Can you work these out from the model? Positions are in its coordinate system, mm. Face numbers are marked on the shaded views. A direction names the side the tool comes from. Round coordinates to 2 decimals unless told otherwise and drop trailing zeros. Loops run counter-clockwise (first coordinate to the right, second up) from the corner with the lowest first, then second, coordinate; pieces in that order, holes last. Notation, with made-up numbers: M -12,65.5 L 4,65.5 A33 ccw 4,93.5 Z; hole C 53.25,28 d7. An arc over 180 degrees is marked long. Answer as CSV lines item,"result".
from build123d import *

# Parameters (mm, degrees)
MAINBASESKETCH_W              = 47.8
MAINBASESKETCH_H              = 3.2
MAINBASEEXTRUDE_DEPTH         = 7.9
MAINBASESHELL_T               = -1.2
UNDERSIDECIRCLEEXT_START      = -0.2
UNDERSIDECIRCLESKETCH_R       = 3.25
UNDERSIDECIRCLESKETCH_R_2     = 2.4
UNDERSIDECIRCLEEXT_DEPTH      = 2.4
UNDERSIDECIRCLEPATTERN_COUNT  = 2
UNDERSIDECIRCLEPATTERN_PITCH  = 8
EXTENDEDBASEEDGECUT_DEPTH     = 0.2
EXTENDEDBASEEDGECUT2_DEPTH    = 0.2
EXTENDEDBASEEDGECUT3_DEPTH    = 0.2
EXTENDEDBASEEDGESKETCH4_W     = 47.4
EXTENDEDBASEEDGESKETCH4_H     = 0.199766916
EXTENDEDBASEEDGECUT4_DEPTH    = 0.2
EXTENDEDNBASEUNDERNOTCH_DEPTH = 0.4
EXTENDEBASENOTCHFILLET_R      = 0.2
CUT_EXTRUDE61_DEPTH           = 50.22551315
CUT_EXTRUDE61_DEPTH_BACK      = 50.22551315


with BuildPart() as part:
    # MainBaseSketch → MainBaseExtrude (new, symmetric)
    with BuildSketch(Plane.XY):
        with Locations((24.581967213, 1.6)):
            Rectangle(MAINBASESKETCH_W, MAINBASESKETCH_H)
    extrude(amount=MAINBASEEXTRUDE_DEPTH, both=True)

    # MainBaseShell
    mainbaseshell_openings = [part.faces().sort_by_distance(p)[0] for p in [
        (24.581967213, 0, 0),
    ]]
    offset(amount=MAINBASESHELL_T, openings=mainbaseshell_openings, kind=Kind.INTERSECTION)

    # UnderSideCircleSketch → UnderSideCircleExt (add)
    with BuildSketch(Plane.XZ.offset(-2).offset(UNDERSIDECIRCLEEXT_START)):
        with Locations((8.581967213, 0)):
            Circle(UNDERSIDECIRCLESKETCH_R)
        with Locations((8.581967213, 0)):
            Circle(UNDERSIDECIRCLESKETCH_R_2, mode=Mode.SUBTRACT)
    undersidecircleext = extrude(amount=UNDERSIDECIRCLEEXT_DEPTH)

    # UnderSideCirclePattern: UnderSideCircleExt ×2
    with Locations(*[(i * UNDERSIDECIRCLEPATTERN_PITCH, 0, 0) for i in range(1, UNDERSIDECIRCLEPATTERN_COUNT)]):
        add(undersidecircleext)

    # ExtendedBaseEdgeSketch → ExtendedBaseEdgeCut (cut)
    with BuildSketch(Plane.ZY.offset(-0.681967213)):
        Polygon((-7.9, 0), (-7.9, 0.199766916), (-7.702184024, 0.199766916), (7.702184024, 0.199766916), (7.9, 0.199766916), (7.9, 0), (7.702184024, 0), (-7.702184024, 0), align=None)
    extrude(amount=-EXTENDEDBASEEDGECUT_DEPTH, mode=Mode.SUBTRACT)

    # ExtendedBaseEdgeSketch2 → ExtendedBaseEdgeCut2 (cut)
    with BuildSketch(Plane(origin=(0, 0, -7.9), x_dir=(-1, 0, 0), z_dir=(0, 0, -1))):
        Polygon((-48.481967213, 0), (-48.481967213, 0.203418418), (-0.881967213, 0.199766916), (-0.881967213, 0), align=None)
    extrude(amount=-EXTENDEDBASEEDGECUT2_DEPTH, mode=Mode.SUBTRACT)

    # ExtendedBaseEdgeSketch3 → ExtendedBaseEdgeCut3 (cut)
    with BuildSketch(Plane(origin=(48.481967213, 0, 0), x_dir=(0, 0, -1), z_dir=(1, 0, 0))):
        Polygon((-7.9, 0), (-7.9, 0.199766916), (7.7, 0.203418418), (7.7, 0), align=None)
    extrude(amount=-EXTENDEDBASEEDGECUT3_DEPTH, mode=Mode.SUBTRACT)

    # ExtendedBaseEdgeSketch4 → ExtendedBaseEdgeCut4 (cut)
    with BuildSketch(Plane.XY.offset(7.9)):
        with Locations((24.581967213, 0.099883458)):
            Rectangle(EXTENDEDBASEEDGESKETCH4_W, EXTENDEDBASEEDGESKETCH4_H)
    extrude(amount=-EXTENDEDBASEEDGECUT4_DEPTH, mode=Mode.SUBTRACT)

    # ExtendedbaseUnderNotchSketch → ExtendednbaseUnderNotch (cut)
    with BuildSketch(Plane.XZ.offset(-2)):
        Polygon((1.881967213, 0), (1.881967213, 2.502100162), (2.381942481, 2.502100162), (2.381942481, -2.499482153), (1.881967213, -2.499482153), align=None)
    extrude(amount=-EXTENDEDNBASEUNDERNOTCH_DEPTH, mode=Mode.SUBTRACT)

    # ExtendebaseNotchFillet
    extendebasenotchfillet_edges = [part.edges().sort_by_distance(p)[0] for p in [
        (1.881967213, 2.4, 0.001309004),
        (2.131954847, 2.4, 2.502100162),
        (2.381942481, 2.4, 0.001309004),
        (2.131954847, 2.4, -2.499482153),
    ]]
    fillet(extendebasenotchfillet_edges, radius=EXTENDEBASENOTCHFILLET_R)

    # Sketch180 → Cut-Extrude61 (cut, two sides: drawn at the far end of the back side and taken through both)
    with BuildSketch(Plane(origin=(0, 0, 0), x_dir=(-1, 0, 0), z_dir=(0, -1, 0)).offset(-CUT_EXTRUDE61_DEPTH_BACK)):
        Polygon((-48.481967213, 7.9), (-24.493136363, 7.9), (-24.481967213, -7.9), (-48.481967213, -7.9), align=None)
    extrude(amount=CUT_EXTRUDE61_DEPTH + CUT_EXTRUDE61_DEPTH_BACK, mode=Mode.SUBTRACT)

    # Sweep30: sweep along a curve in space
    with BuildLine() as sweep30_path:
        Line((24.492288074, 0, -6.7), (24.492288074, 2, -6.7))
    # Sketch181 → Sweep30 (sweep)
    with BuildSketch(Plane(origin=(0, 0, 0), x_dir=(-1, 0, 0), z_dir=(0, -1, 0))):
        Polygon((-24.492288074, 6.7), (-23.292288074, 6.7), (-23.292288074, -6.7), (-24.482815503, -6.7), align=None)
    sweep(path=sweep30_path.line)


solid = part.part
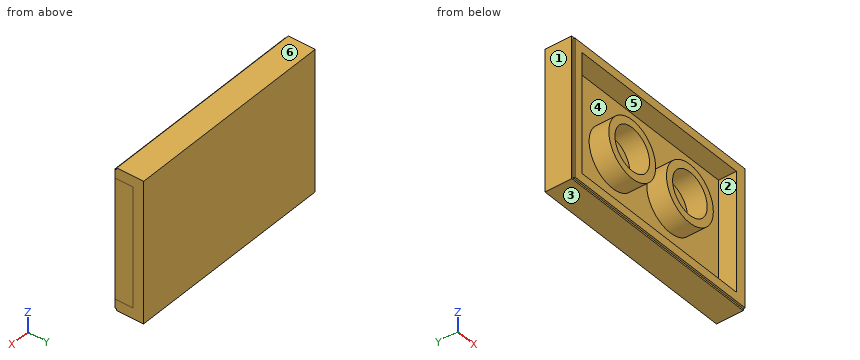
Item 1: On a 3-axis mill with a long thin cutter (end or side, diameter ignored), from which of +Z, -Z, +X, -X, +Y, -Y can I reach the whole of each face in a straight line? I mean the marked faces 5 and 6. Say none if no direction works.
Output:
face 5,"-Y"
face 6,"+Z, +X, -X, +Y, -Y"
Item 2: If we section it at B-B on x = 17: Write out the boundary of the cut face in (y, z).
Output:
outline,"M -0.2,-3.22 L 2,-3.22 L 2,-6.7 L 0,-6.7 L 0,-7.7 L 0.2,-7.7 L 0.2,-7.9 L 3.2,-7.9 L 3.2,7.9 L 0.2,7.9 L 0.2,7.7 L 0,7.7 L 0,6.7 L 2,6.7 L 2,3.22 L -0.2,3.22 L -0.2,2.36 L 2,2.36 L 2,-2.36 L -0.2,-2.36 Z"
Item 3: If I drill on line 1 along X through (y, z) = (0.55, 0); line 2 along X through (y, z) = (0.15, -4.25); line 3 along X through (y, z) = (1.5, -6.5), over which ranges is the centre line in solid material (lowest first)? Write a range as from..to.
Output:
line 1,"x = 0.68..1.88, 5.33..6.18, 10.98..11.83, 13.33..14.18, 18.98..19.83, 23.29..24.49"
line 2,"x = 0.88..1.88, 23.29..24.49"
line 3,"x = 0.68..1.88, 23.29..24.49"
Item 4: Will these pins go through, and if not, where does the flat tip stop? pin 1 (3 mm diameter, centred on x = 8.58, z = 0, fed in from -Y); pin 2 (1.5 mm diameter, centred on y = 1.5, z = 3.5, fed in from +X).
Output:
pin 1,"stops at y = 2"
pin 2,"stops at x = 24.49"
Item 5: If we section it at C-C on z = -4: Write out the boundary of the cut face in (x, y).
Output:
outline,"M 0.68,0.2 L 0.88,0.2 L 0.88,0 L 1.88,0 L 1.88,2 L 23.29,2 L 23.29,0 L 24.49,0 L 24.49,3.2 L 0.68,3.2 Z"
Item 6: We'd pull the mould along X, two halves only. Please class the marked faces 1, 2, 3 and 4: released by +X, released by -X, zero draft, split by the parting line, or undercut.
Output:
face 1,"released by -X"
face 2,"undercut"
face 3,"zero draft"
face 4,"undercut"
Item 7: If we section it at A-A on z = 4.25: Write out the boundary of the cut face in (x, y).
Output:
outline,"M 0.68,0.2 L 0.88,0.2 L 0.88,0 L 1.88,0 L 1.88,2 L 23.29,2 L 23.29,0 L 24.48,0 L 24.48,3.2 L 0.68,3.2 Z"
